from build123d import *

# Parameters (mm, degrees)
PAD_DEPTH = 5.5


with BuildPart() as part:
    # Sketch (on Sketch) → Pad (new body, symmetric)
    with BuildSketch(Plane(origin=(0, 0, 0), x_dir=(1, 0, 0), z_dir=(0, 1, 0))):
        with BuildLine():
            Line((-4.3, 0), (-4.3, 14))
            Line((-4.3, 14), (-3, 14))
            Line((-3, 14), (-3, 12))
            Line((-3, 12), (3, 12))
            Line((3, 12), (3, 14))
            Line((3, 14), (4.3, 14))
            Line((4.3, 14), (4.3, 0))
            Line((4.3, 0), (5.5, 0))
            Line((5.5, 0), (5.5, 14))
            ThreePointArc((5.5, 14), (5.207107, 14.707107), (4.5, 15))
            Line((4.5, 15), (-4.5, 15))
            ThreePointArc((-4.5, 15), (-5.207107, 14.707107), (-5.5, 14))
            Line((-5.5, 14), (-5.5, 0))
            Line((-5.5, 0), (-4.3, 0))
        make_face()
    extrude(amount=PAD_DEPTH, both=True)


solid = part.part
Input: part model. Units: mm. Frame: model coordinates. A direction names the side the tool comes from. Round coordinates to 2 decimals unless told otherwise and drop trailing zeros. Loops run counter-clockwise (first coordinate to the right, second up) from the corner with the lowest first, then second, coordinate; pieces in that order, holes last. Notation, with made-up numbers: (-23.5, 50.5) -> (32.5, 50.5) arc R15 cw to (32.5, 76.5) -> close; hole circle Ø10 at (64.5, 77). An arc over 180 degrees is marked (long way). Answer as a JSON object with one key per item and string values. Group by question number.
1) Section query B-B on y = 4.25. Output: boundary loops of the cut face in (x, z).
2) Section query D-D on x = -0.25. Output: boundary loops of the cut face in (y, z).
3) Reachability of faces 1 (the flat face through (0, -5.5, -13)), 2 (the flat face through (0, 0, -12)) from +Z, -Z, +X, -X, +Y, -Y: full face, straight path, thin tool, end or side. Return the list, or none.
4) Section query C-C on x = 4. Output: boundary loops of the cut face in (y, z).
5) Pin query (flat end, axial travel): pin 1 (1.5 mm diameter, centred on x = 3.5, y = 2, fed in from +Z); pin 2 (0.6 mm diameter, centred on x = 3.5, y = -2, fed in from +Z); pin 3 (1.5 mm diameter, centred on x = -1, z = -11, fed in from -Y). Return the tip coordinate at first contact, or that it passes through.
6) Section query A-A on z = -6.25. Output: boundary loops of the cut face in (x, y).
7) Ray query, L1, parallel to X at y = -2.25, z = -8; L2, parallel to X at y = 0.25, z = -13.25; L3, parallel to Z at x = 0.25, y = -1. Return the intervals inside material, ascending.
Reply:
{
 "1": {"outline": "(-5.5, -14) arc R1 ccw to (-4.5, -15) -> (4.5, -15) arc R1 ccw to (5.5, -14) -> (5.5, 0) -> (4.3, 0) -> (4.3, -14) -> (3, -14) -> (3, -12) -> (-3, -12) -> (-3, -14) -> (-4.3, -14) -> (-4.3, 0) -> (-5.5, 0) -> close"},
 "2": {"outline": "(-5.5, -15) -> (5.5, -15) -> (5.5, -12) -> (-5.5, -12) -> close"},
 "3": {"face 1": "+Z, -Z, +X, -X, -Y", "face 2": "+Z, +Y, -Y"},
 "4": {"outline": "(-5.5, -15) -> (5.5, -15) -> (5.5, -14) -> (-5.5, -14) -> close"},
 "5": {"pin 1": "stops at z = -12", "pin 2": "stops at z = -14", "pin 3": "passes through"},
 "6": {"outline": "(-5.5, -5.5) -> (-4.3, -5.5) -> (-4.3, 5.5) -> (-5.5, 5.5) -> close; (4.3, -5.5) -> (5.5, -5.5) -> (5.5, 5.5) -> (4.3, 5.5) -> close"},
 "7": {"L1": "x = -5.5 to -4.3, 4.3 to 5.5", "L2": "x = -5.5 to -4.3, -3 to 3, 4.3 to 5.5", "L3": "z = -15 to -12"}
}
